```python
from build123d import *

# Parameters (mm, degrees)
SKETCH_1_W          = 120
SKETCH_1_H          = 80
EXTRUDE_1_DEPTH     = 50
SKETCH_2_W          = 104
SKETCH_2_H          = 64
CUT_EXTRUDE_1_DEPTH = 42
FILLET_1_R          = 3


with BuildPart() as part:
    # 草图1 → 凸台-拉伸1 (new body)
    with BuildSketch(Plane(origin=(0, 0, 0), x_dir=(1, 0, 0), z_dir=(0, 1, 0))):
        Rectangle(SKETCH_1_W, SKETCH_1_H)
    extrude(amount=EXTRUDE_1_DEPTH)

    # 草图2 → 切除-拉伸1 (cut)
    with BuildSketch(Plane(origin=(0, 50, 0), x_dir=(1, 0, 0), z_dir=(0, 1, 0))):
        Rectangle(SKETCH_2_W, SKETCH_2_H)
    extrude(amount=-CUT_EXTRUDE_1_DEPTH, mode=Mode.SUBTRACT)

    # 圆角1
    fillet_1_edges = [part.edges().sort_by_distance(p)[0] for p in [
        (60, 50, 0),
        (0, 50, -40),
        (-52, 50, 0),
        (0, 50, 32),
        (52, 50, 0),
        (0, 50, -32),
        (-60, 50, 0),
        (0, 50, 40),
    ]]
    fillet(fillet_1_edges, radius=FILLET_1_R)


solid = part.part
```
Source: CAD feature listing. Evaluate the final solid. Frame: model axes, mm. A direction names the side the tool comes from. Coordinates: 2 decimals unless noted, no trailing zeros. Write each loop counter-clockwise with the first axis right and the second up, starting at its lowest first coordinate (ties: lowest second). Pieces come first, ordered by that corner, then holes. Notation, with made-up numbers: M 6,-31.75 L 58,-31.75 A19 ccw 58,-26.75 Z; hole C -18,57.25 d10. An arc over 180 degrees is marked long. Answer as a JSON object with one key per item and string values.
1. Access query for faces 4 (the cylindrical face through (-59.14, 49.1, -0.56)), 5 (the cylindrical face through (0.77, 49.14, 32.9)). Directions: +Z, -Z, +X, -X, +Y, -Y. A direction counts if a zero-diameter tool reaches every point of the face in a straight line with its end or side. Return the directions, or none.
Evaluation:
{"face 4": "+Z, -Z, -X, +Y", "face 5": "+Y"}
2. Cut plane A-A on y = 37. Output: boundary loops of the cut face in (x, z).
Evaluation:
{"outline": "M -60,-40 L 60,-40 L 60,40 L -60,40 Z; hole M -52,-32 L 52,-32 L 52,32 L -52,32 Z"}
3. Draft query along Z for faces 1 (the cylindrical face through (0.84, 49.1, 39.14)), 2 (the cylindrical face through (0.77, 49.14, -32.9)), 3 (the flat face through (60, 23, 1)). Return one class per face: released by +Z, released by -Z, zero draft, split by the parting line, or undercut.
Evaluation:
{"face 1": "released by +Z", "face 2": "undercut", "face 3": "zero draft"}
4. Cut plane C-C on z = 1.5. Output: boundary loops of the cut face in (x, y), plus the area to 3 significant figures.
Evaluation:
{"outline": "M -60,0 L 60,0 L 60,47 A3 ccw 57,50 L 55,50 A3 ccw 52,47 L 52,8 L -52,8 L -52,47 A3 ccw -55,50 L -57,50 A3 ccw -60,47 Z", "area": "1,620 mm^2"}
5. Cut plane B-B on x = 38.5. Output: boundary loops of the cut face in (y, z), plus the area to 3 significant figures.
Evaluation:
{"outline": "M 0,-40 L 47,-40 A3 ccw 50,-37 L 50,-35 A3 ccw 47,-32 L 8,-32 L 8,32 L 47,32 A3 ccw 50,35 L 50,37 A3 ccw 47,40 L 0,40 Z", "area": "1,300 mm^2"}
6. Ray query, L1, parallel to Z at x = 39, y = 9; L2, parallel to X at y = 29, z = -1; L3, parallel to Y at x = 18, z = -27. Return the intervals inside material, ascending.
Evaluation:
{"L1": "-40 to -32, 32 to 40", "L2": "-60 to -52, 52 to 60", "L3": "0 to 8"}
7. Contact query for a flat-ended pin moving along its axis: P1, Ø4, axis at x = 6, z = -8.5, coming from the +Y side. Output: stop coordinate, or through.
Evaluation:
{"P1": "y = 8"}
